from build123d import *

# Parameters (mm, degrees)
F0_W      = 520.7
F0_H      = 127
F1_DEPTH  = 19.05
F3_DEPTH  = 311.15
F5_W      = 520.7
F5_H      = 120.65
F6_DEPTH  = 19.05
F7_W      = 501.65
F7_H      = 6.35
F8_DEPTH  = 6.35
F9_W      = 501.65
F9_H      = 6.35
F10_DEPTH = 317.5


with BuildPart() as f1:
    # F0 (on Front) → F1 (new body)
    with BuildSketch(Plane.XZ):
        Rectangle(F0_W, F0_H)
    extrude(amount=-F1_DEPTH)

    # F2 (on face) → F3 (join)
    with BuildSketch(Plane(origin=(0, 19.05, 0), x_dir=(-1, 0, 0), z_dir=(0, 1, 0))):
        Polygon((-260.35, 57.15), (-260.35, -63.5), (-241.3, -63.5), (-241.3, -57.15), (-250.825, -57.15), (-250.825, -50.8), (-241.3, -50.8), (-241.3, 57.15), align=None)
    extrude(amount=F3_DEPTH)

    # F4: F1 across plane


with BuildPart() as f1_1:
    add(f1.part)
    add(f1.part.mirror(Plane.YZ))

    # F5 (on face) → F6 (join)
    with BuildSketch(Plane(origin=(0, 330.2, 0), x_dir=(-1, 0, 0), z_dir=(0, 1, 0))):
        with Locations((0, -3.175)):
            Rectangle(F5_W, F5_H)
    extrude(amount=F6_DEPTH)

    # F7 (on face) → F8 (cut)
    with BuildSketch(Plane.XZ.offset(-330.2)):
        with Locations((0, -53.975)):
            Rectangle(F7_W, F7_H)
    extrude(amount=-F8_DEPTH, mode=Mode.SUBTRACT)

    # F9 (on face) → F10 (join, through all)
    with BuildSketch(Plane(origin=(0, 19.05, 0), x_dir=(-1, 0, 0), z_dir=(0, 1, 0))):
        with Locations((0, -53.975)):
            Rectangle(F9_W, F9_H)
    extrude(amount=F10_DEPTH)


solid = f1_1.part
CAD build for the part. Positions are in the model's coordinates, mm. A direction names the side the tool comes from. Coordinates: 2 decimals unless noted, no trailing zeros. Write each loop counter-clockwise with the first axis right and the second up, starting at its lowest first coordinate (ties: lowest second). Pieces come first, ordered by that corner, then holes. Notation, with made-up numbers: (7.25, 61) - (28.25, 61) arc R21 ccw to (28.25, 70) - close; hole circle Ø2 at (3, 8). An arc over 180 degrees is marked (long way). Use a Markdown table: item, result. Add a question column.
Item 1: Drill centre lines: L1, parallel to Y at x = 208, z = -20; L2, parallel to X at y = 282, z = 39.5; L3, parallel to Z at x = -124, y = 30. Where is each one in solid material? Low to high. Write a range as from..to.
Item 2: Flat gauge pins, fed straight in: pin 1 (5 mm diameter, centred on x = -105, z = -60, fed in from -Y); pin 2 (6 mm diameter, centred on x = 105.5, y = 236.5, fed in from +Z). Where does each tip first touch, or does it go through?
Item 3: 3-axis set-ups, long thin cutter, end or side, ignore diameter. For faces 4 (the face through (3, 330.2, 4)), 5 (the face through (4, 349.25, -2)), 6 (the face through (3, 172, -57.15)), 7 (the face through (1, 342, 57.15)): which of +Z, -Z, +X, -X, +Y, -Y reach the whole face in a straight line?
Item 4: Band-saw the part on B-B, the plane y = 162.5. Give the cut face in (x, z).
Item 5: Mould opens along X. For faces 1 (the face through (260.35, 172, -1)), 2 (the face through (-4, 0, 1)), 3 (the face through (-241.3, 172, 2)) say: pulls with the +X half, pulls with the -X half, needs draft (parallel to the pull), parting line crosses it, or undercut.
Item 6: Band-saw the part on C-C, the plane x = -215.5. Give the cut face in (y, z), and give its area (3 significant figures).
Item 7: Band-saw the part on A-A, the plane z = 32. Give the cut face in (x, y).
Numbers:
| question | item | result |
|---|---|---|
| 1 | L1 | 0..19.05, 330.2..349.25 |
| 1 | L2 | -260.35..-241.3, 241.3..260.35 |
| 1 | L3 | -57.15..-50.8 |
| 2 | pin 1 | y = 0 |
| 2 | pin 2 | z = -50.8 |
| 3 | face 4 | +Z |
| 3 | face 5 | +Z, -Z, +X, -X, +Y |
| 3 | face 6 | -Z |
| 3 | face 7 | +Z, +X, -X, +Y |
| 4 | outline | (-260.35, -63.5) - (-241.3, -63.5) - (-241.3, -57.15) - (241.3, -57.15) - (241.3, -63.5) - (260.35, -63.5) - (260.35, 57.15) - (241.3, 57.15) - (241.3, -50.8) - (-241.3, -50.8) - (-241.3, 57.15) - (-260.35, 57.15) - close |
| 5 | face 1 | pulls with the +X half |
| 5 | face 2 | needs draft |
| 5 | face 3 | undercut |
| 6 | outline | (0, -63.5) - (19.05, -63.5) - (19.05, -57.15) - (330.2, -57.15) - (330.2, -63.5) - (349.25, -63.5) - (349.25, 57.15) - (330.2, 57.15) - (330.2, -50.8) - (19.05, -50.8) - (19.05, 63.5) - (0, 63.5) - close |
| 6 | area | 6,690 mm2 |
| 7 | outline | (-260.35, 0) - (260.35, 0) - (260.35, 349.25) - (-260.35, 349.25) - close; hole (-241.3, 19.05) - (241.3, 19.05) - (241.3, 330.2) - (-241.3, 330.2) - close |
